from build123d import *


with BuildPart() as part:
    # Sketch2 → Revolve1 (revolve)
    with BuildSketch(Plane.XY, mode=Mode.PRIVATE) as revolve1_sk:
        with BuildLine():
            Line((27.530975966, 168), (27.530975966, 7))
            ThreePointArc((27.530975966, 7), (24.005991012, 4.779859802), (20, 3.636803621))
            Line((20, 3.636803621), (0, 3.636803621))
            Line((0, 3.636803621), (0, 0))
            Line((0, 0), (23, 0))
            ThreePointArc((23, 0), (27.949747468, 2.050252532), (30, 7))
            Line((30, 7), (30, 168))
            Line((30, 168), (27.530975966, 168))
        make_face()
    revolve(revolve1_sk.sketch.rotate(Axis((0, 0, 0), (0, 1, 0)), 90), axis=Axis((0, 0, 0), (0, 1, 0)))


solid = part.part
Build history of the part. All positions in model axes, mm. A direction names the side the tool comes from. Round coordinates to 2 decimals unless told otherwise and drop trailing zeros. Order: outer loops, then holes, each group sorted by start corner. A loop starts at its lowest first (then second) coordinate and runs counter-clockwise, first axis right, second up. Notation, with made-up numbers: M 31.25,32 L 81.25,32 A14 ccw 81.25,53 Z; hole C -39,-39.75 d2. An arc over 180 degrees is marked long. Use CSV: the item, a comma, the result in double quotes. Start each with the question number.
(1) Cut at A-A on x = 0. List the corners of the cut face in (y, z), then the cut area to 3 significant figures.
(2) Drill centre lines: probe 1 along X at (y, z) = (135.5, 0); probe 2 along Y at (x, z) = (15, 5); probe 3 along X at (y, z) = (150, -14.5). Where is each one in solid material? Low to high.
(3) Mould opens along X. For faces 1 (the face through (-25.296, 88.627, -16.128)), 2 (the face through (0, 0, 0)), 3 (the face through (-8.27, 86.37, -26.26)) say: +X half, -X half, draft (parallel to the pull), parting line (faces both ways), or undercut.
(4) Cut at C-C on y = 52. List the corners of the cut face in (x, z).
(5) Cut at B-B on z = 0. List the corners of the cut face in (x, y).
(6) Flat gauge pins, fed straight in: P1, Ø1, axis at y = 92, z = 11.5, coming from the -X side; P2, Ø6, axis at y = 53.5, z = 11.5, coming from the +X side; P3, Ø1.5, axis at y = 43.5, z = 12.5, coming from the -X side. Where does each tip first touch, or does it go through?
(7) Tool access for faces 4 (the face through (27, 168, -9)), 5 (the face through (0, 3.637, 0)): list every direction of +Z, -Z, +X, -X, +Y, -Y with a clear straight run to the whole face (end or side of a thin tool).
Findings:
1,outline,"M 0,-23 A7 ccw 7,-30 L 168,-30 L 168,-27.53 L 7,-27.53 A14.71 cw 3.64,-20 L 3.64,20 A14.71 cw 7,27.53 L 168,27.53 L 168,30 L 7,30 A7 ccw 0,23 Z"
1,area,"1,030 mm^2"
2,probe 1,"x = -30 to -27.53, 27.53 to 30"
2,probe 2,"y = 0 to 3.64"
2,probe 3,"x = -26.26 to -23.4, 23.4 to 26.26"
3,face 1,"parting line"
3,face 2,"draft"
3,face 3,"undercut"
4,outline,"C 0,0 d60; hole C 0,0 d55.06"
5,outline,"M -30,7 A7 ccw -23,0 L 23,0 A7 ccw 30,7 L 30,168 L 27.53,168 L 27.53,7 A14.71 cw 20,3.64 L -20,3.64 A14.71 cw -27.53,7 L -27.53,168 L -30,168 Z"
6,P1,"stops at x = -27.91"
6,P2,"stops at x = 28.77"
6,P3,"stops at x = -27.6"
7,face 4,"+Z, -Z, +X, -X, +Y"
7,face 5,"+Y"
